For this review, use the dimensioned drawing (mm, ordinates from the lowest corner) and the shaded views. A direction names the side the tool comes from. Coordinates: 2 decimals unless noted, no trailing zeros. Order: outer loops, then holes, each group sorted by start corner. A loop starts at its lowest first (then second) coordinate and runs counter-clockwise, first axis right, second up. Notation, with made-up numbers: M -17,27.25 L 11,27.25 A33 ccw 11,61.25 Z; hole C 11,61.5 d3. An arc over 180 degrees is marked long. Answer in a Markdown table with one row per item.
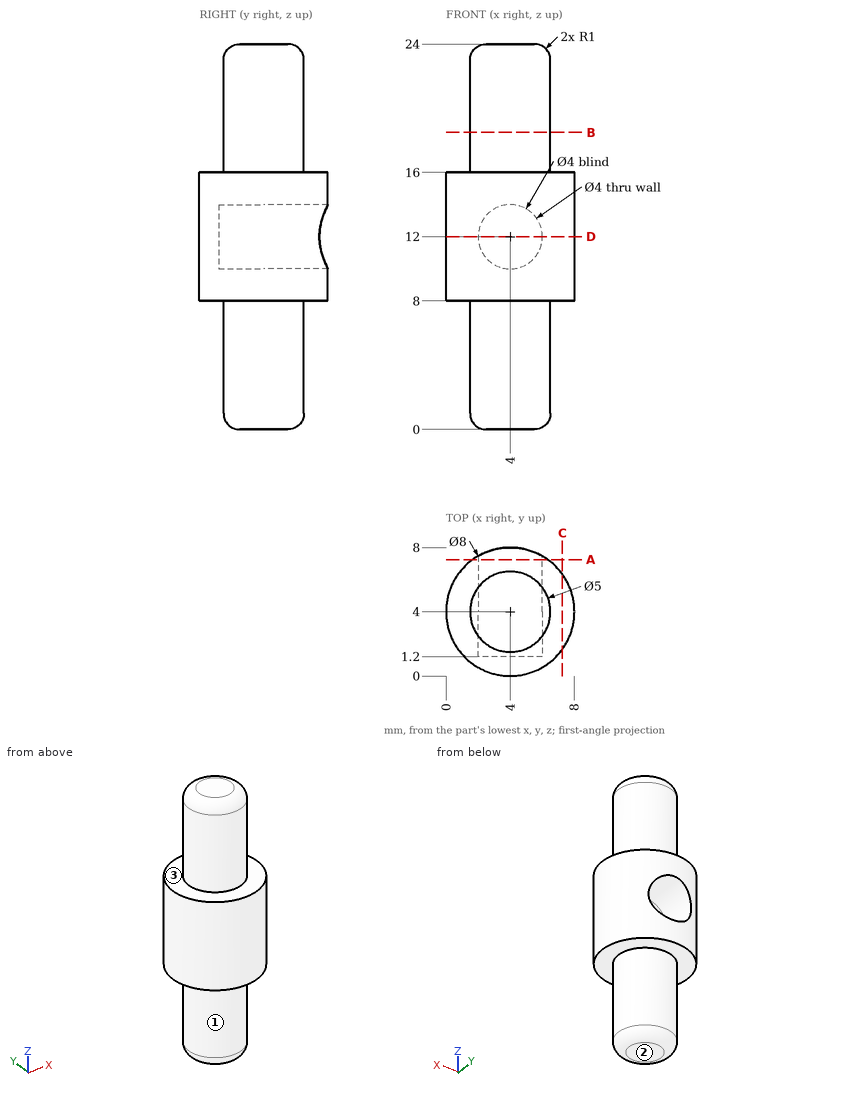
(1) Add section D-D, the plane z = 12. Give the boundary of the cut face in (x, y).
Return value:
| item | result |
|---|---|
| outline | M 2,1.2 L 2,7.46 A4 ccw long 6,7.46 L 6,1.2 Z |
(2) Insertion check: pin 1 Ø2 at (y, z) = (5.5, 20.5) entering from -X; pin 2 Ø4 at (x, z) = (4, 4.5) entering from +Y; pin 3 Ø2 at (y, z) = (4, 4) entering from -X. Each pin has a flat end and moves straight along its axis. Give the tip position at first contact, or say it passes through.
Return value:
| item | result |
|---|---|
| pin 1 | stops at x = 1.55 |
| pin 2 | stops at y = 6.5 |
| pin 3 | stops at x = 1.5 |
(3) For line 1 along Z through (x, y) = (4, 3.25); line 2 along Z through (x, y) = (5.75, 0.5); line 3 along Z through (x, y) = (2.5, 7.25), list the stretches that pass through material, from the lowest coordinate up. Write a range as from..to.
Return value:
| item | result |
|---|---|
| line 1 | z = 0..10, 14..24 |
| line 2 | z = 8..16 |
| line 3 | z = 8..10.68, 13.32..16 |
(4) Add section B-B, the plane z = 18.5. Give the boundary of the cut face in (x, y).
Return value:
| item | result |
|---|---|
| outline | C 4,4 d5 |
(5) For the marked faces 1, 2 and 3, list the 3-axis set-ups (+Z, -Z, +X, -X, +Y, -Y) from which the entire face can be reached by the end or side of a thin tool; tool diameter is ignored.
Return value:
| item | result |
|---|---|
| face 1 | -Z |
| face 2 | -Z, +X, -X, +Y, -Y |
| face 3 | +Z |
(6) Add section C-C, the plane x = 7.25. Give the boundary of the cut face in (y, z).
Return value:
| item | result |
|---|---|
| outline | M 1.67,8 L 6.33,8 L 6.33,16 L 1.67,16 Z |
(7) Add section A-A, the plane y = 7.25. Give the boundary of the cut face in (x, z), and give its area (3 significant figures).
Return value:
| item | result |
|---|---|
| outline | M 1.67,8 L 6.33,8 L 6.33,16 L 1.67,16 Z; hole C 4,12 d4 |
| area | 24.7 mm2 |
